Model file for the job. Use its own axes, mm. A direction names the side the tool comes from. Coordinates: 2 decimals unless noted, no trailing zeros. Order: outer loops, then holes, each group sorted by start corner. A loop starts at its lowest first (then second) coordinate and runs counter-clockwise, first axis right, second up.
from build123d import *

# Parameters (mm, degrees)
EXTRUSION1_DEPTH = 42
ESQUISSE2_R      = 1.5
EXTRUSION2_DEPTH = 49.350239901
ESQUISSE3_R      = 1.5
EXTRUSION3_DEPTH = 10
ESQUISSE4_R      = 11.5
EXTRUSION4_DEPTH = 10
ESQUISSE5_R      = 3
EXTRUSION5_DEPTH = 10


with BuildPart() as part:
    # Esquisse1 → Extrusion1 (new body)
    with BuildSketch(Plane.XY):
        Polygon((-15.613581117, 13.181263158), (-15.613581117, -6.818736842), (4.386418883, -6.818736842), (4.386418883, 13.181263158), (2.886418883, 13.181263158), (2.886418883, -5.318736842), (-14.113581117, -5.318736842), (-14.113581117, 13.181263158), align=None)
    extrude(amount=EXTRUSION1_DEPTH)

    # Esquisse2 → Extrusion2 (cut, through all)
    with BuildSketch(Plane(origin=(4.386418883, 0, 0), x_dir=(0, 0, -1), z_dir=(1, 0, 0))):
        with Locations((-36.5, -2.318736842)):
            Circle(ESQUISSE2_R)
        with Locations((-5.5, -2.318736842)):
            Circle(ESQUISSE2_R)
    extrude(amount=-EXTRUSION2_DEPTH, mode=Mode.SUBTRACT)

    # Esquisse3 → Extrusion3 (cut)
    with BuildSketch(Plane(origin=(4.386418883, 0, 0), x_dir=(0, 0, -1), z_dir=(1, 0, 0))):
        with Locations((-21, -2.318736842)):
            Circle(ESQUISSE3_R)
    extrude(amount=-EXTRUSION3_DEPTH, mode=Mode.SUBTRACT)

    # Esquisse4 → Extrusion4 (cut)
    with BuildSketch(Plane.ZY.offset(15.613581117)):
        with Locations((21, 13.181263158)):
            Circle(ESQUISSE4_R)
    extrude(amount=-EXTRUSION4_DEPTH, mode=Mode.SUBTRACT)

    # Esquisse5 → Extrusion5 (cut)
    with BuildSketch(Plane(origin=(4.386418883, 0, 0), x_dir=(0, 0, -1), z_dir=(1, 0, 0))):
        with Locations((-21, 13.181263158)):
            Circle(ESQUISSE5_R)
    extrude(amount=-EXTRUSION5_DEPTH, mode=Mode.SUBTRACT)


solid = part.part
Q1. Drop a flat-ended pin along its axis: P1, Ø8.5, axis at x = -3, z = 16.5, coming from the +Y side. Give the stop position or say it passes through.
Established:
P1: stops at y = -5.32
Q2. Which spindle directions (+Z, -Z, +X, -X, +Y, -Y) get a long thin tool onto all of the face, cutting with end or side? Do faces 1 (the face through (-5, -5.319, 21)), 2 (the face through (3.6, -2.3, 22.5)), 3 (the face through (-14.874, 1.684, 20.747)), 4 (the face through (-15.614, 1, 21)). Say none if no direction does.
Established:
face 1: +Z, -Z, +Y
face 2: +X
face 3: -X, +Y
face 4: +Z, -Z, -X, +Y, -Y
Q3. Cut at C-C, the plane z = 5.5. List the corners of the cut face in (x, y).
Established:
outline: (-15.61, -6.82) - (4.39, -6.82) - (4.39, -3.82) - (2.89, -3.82) - (2.89, -5.32) - (-14.11, -5.32) - (-14.11, -3.82) - (-15.61, -3.82) - close; (-15.61, -0.82) - (-14.11, -0.82) - (-14.11, 13.18) - (-15.61, 13.18) - close; (2.89, -0.82) - (4.39, -0.82) - (4.39, 13.18) - (2.89, 13.18) - close
Q4. Cut at D-D, the plane y = 6.5. List the corners of the cut face in (x, z), plus the area to 3 significant figures.
Established:
outline: (-15.61, 0) - (-14.11, 0) - (-14.11, 11.64) - (-15.61, 11.64) - close; (-15.61, 30.36) - (-14.11, 30.36) - (-14.11, 42) - (-15.61, 42) - close; (2.89, 0) - (4.39, 0) - (4.39, 42) - (2.89, 42) - close
area: 97.9 mm2
Q5. Cut at A-A, the plane z = 21. List the corners of the cut face in (x, y), plus the area to 4 significant figures.
Established:
outline: (-15.61, -6.82) - (4.39, -6.82) - (4.39, -3.82) - (2.89, -3.82) - (2.89, -5.32) - (-14.11, -5.32) - (-14.11, 1.68) - (-15.61, 1.68) - close; (2.89, -0.82) - (4.39, -0.82) - (4.39, 10.18) - (2.89, 10.18) - close
area: 59.25 mm2
Q6. Mould opens along Z. For faces 5 (the face through (3.65, -3.23, 37.69)), 6 (the face through (-14.85, -3.23, 6.69)), 7 (the face through (-15, 13.181, 5)), 8 (the face through (-6, -6, 0)) say: pulls with the +Z half, pulls with the -Z half, needs draft (parallel to the pull), parting line crosses it, or undercut.
Established:
face 5: undercut
face 6: undercut
face 7: needs draft
face 8: pulls with the -Z half
Q7. Probe line 1 (X direction, y = 10.5, z = 6); line 2 (Y direction, x = -14.8, z = 36.5); line 3 (Y direction, x = -10.75, z = 40.5). List the from-to ranges inside material, lowest first.
Established:
line 1: x = -15.61 to -14.11, 2.89 to 4.39
line 2: y = -6.82 to -3.82, -0.82 to 13.18
line 3: y = -6.82 to -5.32
Q8. Cut at B-B, the plane y = -0.25. List the corners of the cut face in (x, z).
Established:
outline: (-15.61, 0) - (-14.11, 0) - (-14.11, 42) - (-15.61, 42) - close; (2.89, 0) - (4.39, 0) - (4.39, 42) - (2.89, 42) - close
